from build123d import *

# Parameters (mm, degrees)
F0_W     = 25.4
F0_H     = 25.4
F1_DEPTH = 6.35
F3_D     = 8.0264
F5_D     = 3.4544
F5_DEPTH = 15.08125
F5_TIP   = 1.0378064612
F6_SIZE  = 2.54


with BuildPart() as f1:
    # F0 (on Front) → F1 (new body, symmetric)
    with BuildSketch(Plane.XZ):
        with Locations((0, -12.7)):
            Rectangle(F0_W, F0_H)
    extrude(amount=F1_DEPTH, both=True)

    # F3 (through all)
    with Locations(Plane.XZ.offset(6.35)):
        with Locations((0, -12.7)):
            Hole(F3_D / 2)

    # F5
    with Locations(Plane(origin=(0, 0, -25.4), x_dir=(1, 0, 0), z_dir=(0, 0, -1))):
        with Locations((0, 0)):
            Hole(F5_D / 2, depth=F5_DEPTH)
            with Locations((0, 0, -(F5_DEPTH + F5_TIP / 2))):  # 118° drill point
                Cone(0, F5_D / 2, F5_TIP, mode=Mode.SUBTRACT)

    # F6
    f6_edges = [f1.edges().sort_by_distance(p)[0] for p in [
        (12.7, 0, -25.4),
        (-12.7, 0, -25.4),
        (-12.7, 0, 0),
        (12.7, 0, 0),
    ]]
    chamfer(f6_edges, length=F6_SIZE)


solid = f1.part
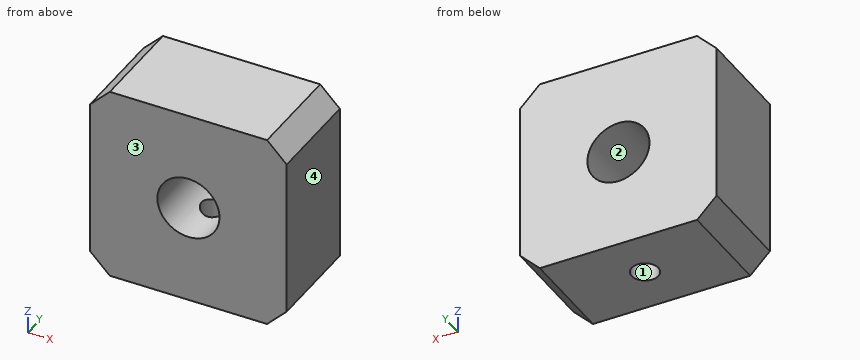
Model file for the job. Use its own axes, mm. Face numbers are marked on the shaded views. Give positions to 0.01 mm unless a question says otherwise; leave off trailing zeros. Loops run counter-clockwise (first coordinate to the right, second up) from the corner with the lowest first, then second, coordinate; pieces in that order, holes last.
1) Pull direction X, two halves, no side cores. Call the marked faces 1, 2, 3 and 4: +X half, -X half, draft (parallel to the pull), parting line (faces both ways), or undercut.
2) Wall check: line 1 (Z direction, x = 0, y = 2.25); line 2 (Z direction, x = 3, y = 2); line 3 (Y direction, x = 1.25, z = -21). Give the ranges that are in metal, low to high.
3) Saw through at C-C (x = 0). Write the cut outline in (y, z), plus the area to 3 significant figures.
4) Saw through at D-D (z = -24). Write the cut outline in (x, y), plus the area to 3 significant figures.
5) Saw through at B-B (y = 5.25). Write the cut outline in (x, z), plus the area to 3 significant figures.
6) Saw through at A-A (z = -12.7). Write the cut outline in (x, y), plus the area to 3 significant figures.
Answer block:
1. face 1: undercut
1. face 2: undercut
1. face 3: draft
1. face 4: +X half
2. line 1: z = -25.4 to -16.71, -8.69 to 0
2. line 2: z = -25.4 to -15.37, -10.03 to 0
2. line 3: y = -6.35 to -1.19, 1.19 to 6.35
3. outline: (-6.35, -25.4) - (-1.73, -25.4) - (-1.73, -16.71) - (-6.35, -16.71) - close; (-6.35, -8.69) - (6.35, -8.69) - (6.35, 0) - (-6.35, 0) - close; (1.73, -25.4) - (6.35, -25.4) - (6.35, -16.71) - (1.73, -16.71) - close
3. area: 191 mm2
4. outline: (-11.56, -6.35) - (11.56, -6.35) - (11.56, 6.35) - (-11.56, 6.35) - close; hole circle Ø3.45 at (0, 0)
4. area: 284 mm2
5. outline: (-12.7, -22.86) - (-10.16, -25.4) - (10.16, -25.4) - (12.7, -22.86) - (12.7, -2.54) - (10.16, 0) - (-10.16, 0) - (-12.7, -2.54) - close; hole circle Ø8.03 at (0, -12.7)
5. area: 582 mm2
6. outline: (-12.7, -6.35) - (-4.01, -6.35) - (-4.01, 6.35) - (-12.7, 6.35) - close; (4.01, -6.35) - (12.7, -6.35) - (12.7, 6.35) - (4.01, 6.35) - close
6. area: 221 mm2
